from build123d import *

# Parameters (mm, degrees)
BOSS_EXTRUDE1_DEPTH          = 50.8
F_3_0_3_DIAMETER_HOLE1_D     = 3
F_3_0_3_DIAMETER_HOLE1_DEPTH = 50.8
CHAMFER1_SIZE                = 0.35


with BuildPart() as part:
    # Sketch1 → Boss-Extrude1 (new body)
    with BuildSketch(Plane.XY.offset(50.8)):
        Polygon((-3.579571669, 0), (-1.789785834, -3.1), (1.789785834, -3.1), (3.579571669, 0), (1.789785834, 3.1), (-1.789785834, 3.1), align=None)
    extrude(amount=-BOSS_EXTRUDE1_DEPTH)

    # Ø3.0 (3) Diameter Hole1
    with Locations(Plane.XY.offset(50.8)):
        with Locations((0, 0)):
            Hole(F_3_0_3_DIAMETER_HOLE1_D / 2, depth=F_3_0_3_DIAMETER_HOLE1_DEPTH)

    # Chamfer1
    chamfer1_edges = [part.edges().sort_by_distance(p)[0] for p in [
        (1.5, 0, 50.8),
        (1.5, 0, 0),
    ]]
    chamfer(chamfer1_edges, length=CHAMFER1_SIZE)


solid = part.part
Geometry: final body of the model. Coordinates: model frame, mm. Coordinates: 2 decimals unless noted, no trailing zeros. Write each loop counter-clockwise with the first axis right and the second up, starting at its lowest first coordinate (ties: lowest second). Pieces come first, ordered by that corner, then holes. Notation, with made-up numbers: (49.5, 9) - (84.5, 9) arc R16 cw to (84.5, 37) - close; hole circle Ø3 at (80, 89.25). An arc over 180 degrees is marked (long way). Return JSON: item names as keys, results as strings.
Item 1: Line query: L1, parallel to Y at x = 0, z = 16.5; L2, parallel to X at y = -0.5, z = 45; L3, parallel to Y at x = 1, z = 11.5. Output: solid intervals per line, ascending.
Completed:
{"L1": "y = -3.1 to -1.5, 1.5 to 3.1", "L2": "x = -3.29 to -1.41, 1.41 to 3.29", "L3": "y = -3.1 to -1.12, 1.12 to 3.1"}
Item 2: Pull-direction query (Y, two-part tool) for faces 1 (the face through (0, -3.1, 26)), 2 (the face through (1.5, 0.07, 25.05)), 3 (the face through (2.697, 1.528, 25.756)); classes: +Y half, -Y half, draft (parallel to the pull), parting line (faces both ways), or undercut.
Completed:
{"face 1": "-Y half", "face 2": "undercut", "face 3": "+Y half"}
Item 3: Section query A-A (x = 0). Output: boundary loops of the cut face in (y, z).
Completed:
{"outline": "(-3.1, 0) - (-1.85, 0) - (-1.5, 0.35) - (-1.5, 50.45) - (-1.85, 50.8) - (-3.1, 50.8) - close; (1.5, 0.35) - (1.85, 0) - (3.1, 0) - (3.1, 50.8) - (1.85, 50.8) - (1.5, 50.45) - close"}
Item 4: Section query B-B (z = 22.5). Output: boundary loops of the cut face in (x, y).
Completed:
{"outline": "(-3.58, 0) - (-1.79, -3.1) - (1.79, -3.1) - (3.58, 0) - (1.79, 3.1) - (-1.79, 3.1) - close; hole circle Ø3 at (0, 0)"}
Item 5: Pin query (flat end, axial travel): pin 1 Ø1 at (x, y) = (1.5, -0.5) entering from -Z; pin 2 Ø1 at (y, z) = (1, 34.5) entering from -X. Return the tip coordinate at first contact, or that it passes through.
Completed:
{"pin 1": "stops at z = 0", "pin 2": "stops at x = -3.29"}
Item 6: Section query C-C (x = 3). Output: boundary loops of the cut face in (y, z).
Completed:
{"outline": "(-1, 0) - (1, 0) - (1, 50.8) - (-1, 50.8) - close"}
